Print and shaded views of the part. All mm, measured from the part's lowest x, y and z. A direction names the side the tool comes from. Give positions to 0.01 mm unless a question says otherwise; leave off trailing zeros. Write each loop counter-clockwise with the first axis right and the second up, starting at its lowest first coordinate (ties: lowest second). Pieces come first, ordered by that corner, then holes. Notation, with made-up numbers: M 12,41 L 60,41 A23 ccw 60,61 Z; hole C -9.5,19 d7. An arc over 180 degrees is marked long. One line per question, with ' | ' between items. Start each with the question number.
1. Which spindle directions (+Z, -Z, +X, -X, +Y, -Y) get a long thin tool onto all of the face, cutting with end or side? Do the marked faces 1, 2 and 3. Say none if no direction does.
2. Wall check: L1, parallel to Z at x = 73, y = 7; L2, parallel to Y at x = 64, z = 2; L3, parallel to Y at x = 40, z = 6. Give the ranges that are in metal, low to high.
3. Cut at A-A, the plane y = 49. Write the cut outline in (x, z).
4. Flat gauge pins, fed straight in: pin 1 (5 mm diameter, centred on x = 73, z = 7, fed in from -Y); pin 2 (8 mm diameter, centred on x = 16, y = 8.5, fed in from -Z); pin 3 (10 mm diameter, centred on x = 71, z = 18, fed in from +Y); pin 4 (1.5 mm diameter, centred on x = 56.5, y = 53.5, fed in from +Z). Where does each tip first touch, or does it go through?
5. Pull direction X, two halves, no side cores. Call the marked faces 4, 5, 6 and 7: released by +X, released by -X, zero draft, split by the parting line, or undercut.
6. Cut at C-C, the plane x = 40. Write the cut outline in (y, z).
7. Cut at B-B, the plane y = 16. Write the cut outline in (x, z), then the cut area to 3 significant figures.
8. Cut at D-D, the plane z = 16.5. Write the cut outline in (x, y).
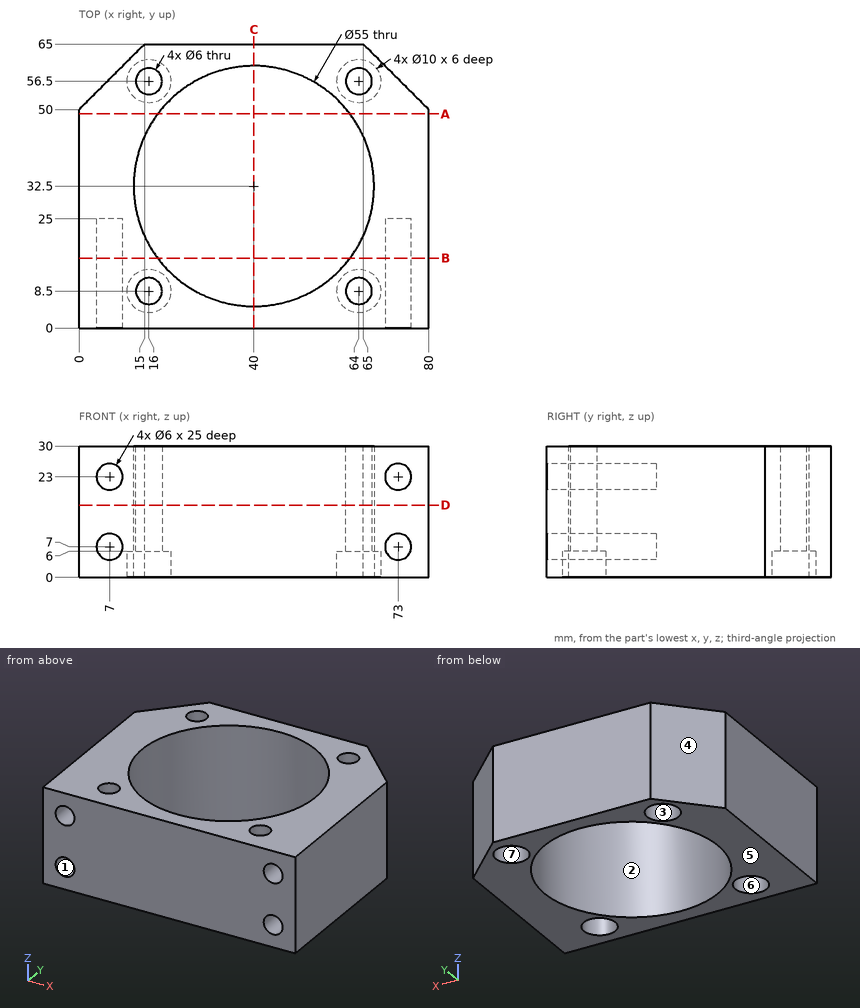
Here are the results:
1) face 1: -Y | face 2: +Z, -Z | face 3: -Z
2) L1: 0 to 4, 10 to 20, 26 to 30 | L2: 0 to 3.5, 13.5 to 19.07, 45.93 to 51.5, 61.5 to 65 | L3: 0 to 5, 60 to 65
3) outline: M 0,0 L 18,0 L 18,30 L 0,30 Z; M 62,0 L 80,0 L 80,30 L 62,30 Z
4) pin 1: y = 25 | pin 2: z = 6 | pin 3: y = 64 | pin 4: through
5) face 4: released by -X | face 5: zero draft | face 6: undercut | face 7: undercut
6) outline: M 0,0 L 5,0 L 5,30 L 0,30 Z; M 60,0 L 65,0 L 65,30 L 60,30 Z
7) outline: M 0,0 L 18,0 L 18,30 L 0,30 Z; M 62,0 L 80,0 L 80,30 L 62,30 Z; hole C 7,7 d6; hole C 7,23 d6; hole C 73,7 d6; hole C 73,23 d6 | area: 967 mm^2
8) outline: M 0,0 L 80,0 L 80,50 L 65,65 L 15,65 L 0,50 Z; hole C 40,32.5 d55; hole C 16,8.5 d6; hole C 16,56.5 d6; hole C 64,8.5 d6; hole C 64,56.5 d6
